from build123d import *

# Parameters (mm, degrees)
EXTRUDE_1_DEPTH     = 16
SKETCH_2_R          = 15.5
CUT_EXTRUDE_2_DEPTH = 649.427486061


with BuildPart() as part:
    # 草图1 → 拉伸1 (new body)
    with BuildSketch(Plane.XY):
        Polygon((-395.537960369, 313.567840296), (-395.537960369, -296.432159704), (-165.537960369, -496.432159704), (-115.537960369, -496.432159704), (29.462039631, -363.432159704), (29.462039631, 380.567840296), (-115.537960369, 513.567840296), (-165.537960369, 513.567840296), align=None)
    extrude(amount=EXTRUDE_1_DEPTH)

    # 草图2 → 拉伸2 (cut, through all)
    with BuildSketch(Plane.XY.offset(16)):
        with Locations((-350.537960369, -51.432159704)):
            Circle(SKETCH_2_R)
        with Locations((-350.537960369, -251.432159704)):
            Circle(SKETCH_2_R)
        with Locations((-350.537960369, -151.432159704)):
            Circle(SKETCH_2_R)
        with Locations((-194.104974179, -264.23694972)):
            Circle(SKETCH_2_R)
        with Locations((-112.77894091, -352.475695817)):
            Circle(SKETCH_2_R)
        with Locations((-98.292741234, -257.527551975)):
            Circle(SKETCH_2_R)
        with Locations(Location((-208.591173855, -359.185093562, 0), (0, 0, 180))):
            Circle(SKETCH_2_R)
        with Locations((-127.265140586, -447.423839658)):
            Circle(SKETCH_2_R)
        with Locations(Location((-16.966707965, -345.766298072, 0), (0, 0, 180))):
            Circle(SKETCH_2_R)
        with Locations((-16.966707965, 362.901978664)):
            Circle(SKETCH_2_R)
        with Locations(Location((-127.265140586, 464.55952025, 0), (0, 0, 180))):
            Circle(SKETCH_2_R)
        with Locations((-208.591173855, 376.320774153)):
            Circle(SKETCH_2_R)
        with Locations(Location((-98.292741234, 274.663232567, 0), (0, 0, 180))):
            Circle(SKETCH_2_R)
        with Locations(Location((-112.77894091, 369.611376409, 0), (0, 0, 180))):
            Circle(SKETCH_2_R)
        with Locations(Location((-194.104974179, 281.372630312, 0), (0, 0, 180))):
            Circle(SKETCH_2_R)
        with Locations(Location((-350.537960369, 168.567840296, 0), (0, 0, 180))):
            Circle(SKETCH_2_R)
        with Locations(Location((-350.537960369, 268.567840296, 0), (0, 0, 180))):
            Circle(SKETCH_2_R)
        with Locations(Location((-350.537960369, 68.567840296, 0), (0, 0, 180))):
            Circle(SKETCH_2_R)
    extrude(amount=-CUT_EXTRUDE_2_DEPTH, mode=Mode.SUBTRACT)


solid = part.part
For this review, take the finished solid that the model builds, in its own axes (mm). Round coordinates to 2 decimals unless told otherwise and drop trailing zeros. Write each loop counter-clockwise with the first axis right and the second up, starting at its lowest first coordinate (ties: lowest second). Pieces come first, ordered by that corner, then holes. Notation, with made-up numbers: (-34.5, 53) - (-3.5, 53) arc R16 cw to (-3.5, 76) - close; hole circle Ø6 at (13.25, 28.5). An arc over 180 degrees is marked (long way). Write item = value, one per line. Start each with the question number.
1. Wall thickness on L1, parallel to Y at x = -99, z = 5.25; L2, parallel to Y at x = -189.5, z = 12.5; L3, parallel to Y at x = -23, z = 5.25: over which ranges is each line inside the solid? List them lowest first.
2. Draft analysis for pull direction X (two halves, no side actions). For faces 1 (the face through (-42.023, 446.137, 7.888)), 2 (the face through (-181.8, 290.8, 8.1)), 3 (the face through (-186, 16, 16)), state which applies: released by +X, released by -X, zero draft, split by the parting line, or undercut.
3. For pin 1 Ø6 at (x, z) = (-86.5, 4) entering from -Y; pin 2 Ø8 at (x, z) = (-44.5, 11) entering from +Y, all flat-tipped, find the tip position at first contact; note any pin that passes through.
4. Consider section A-A on z = 8. Give the number of separate pieces and of enclosed holes in the cut face, plus the area to 3 significant figures.
5. Consider section B-B on x = -317. State the section outline as (y, z) points, plus the area to 3 significant figures.
Evaluation:
q1.L1 = -481.26 to -359.57, -345.38 to -273.01, -242.04 to 259.18, 290.15 to 362.51, 376.71 to 498.4
q1.L2 = -475.6 to -279.04, -249.44 to 266.57, 296.17 to 492.73
q1.L3 = -411.55 to -360.04, -331.49 to 348.62, 377.18 to 428.69
q2.face_1 = released by +X
q2.face_2 = undercut
q2.face_3 = zero draft
q3.pin_1 = -472.55
q3.pin_2 = 452.08
q4.separate_pieces = 1
q4.enclosed_holes = 18
q4.area = 350,000 mm2
q5.outline = (-364.73, 0) - (381.86, 0) - (381.86, 16) - (-364.73, 16) - close
q5.area = 11,900 mm2
